Autodesk Inventor part; units mm, degrees
ref_plane "YZ Plane" through (0, 0, 0) normal (1, 0, 0) x (0, 1, 0)
ref_plane "XZ Plane" through (0, 0, 0) normal (0, 1, 0) x (-1, 0, 0)
ref_plane "XY Plane" through (0, 0, 0) normal (0, 0, 1) x (1, 0, 0)
sketch "DrumSketch" plane through (0, 0, 0) normal (0, 0, 1) x (1, 0, 0)
  line L0 (0, 8.12) -> (0, -9.52)
  line L1 (-7.84, 0) -> (7.84, 0)
  circle A0 centre (0, 0) radius 4.2
  line L2 (-2.7, -3) -> (2.7, -3)
  line L3 (2.7, 0) -> (2.7, -7)
  line L4 (2.7, -7) -> (-2.7, -7)
  line L5 (-2.7, -7) -> (-2.7, 0)
  circle A1 centre (0, 0) radius 5.6
  dimension "d0" = 8.4
  dimension "d1" = 5.4
  dimension "d2" = 7
  dimension "d3" = 4
  dimension "d6" = 11.2
sketch "BodySketch" plane through (0, 0, 0) normal (0, 1, 0) x (-1, 0, 0)
  line L0 (8, 16) -> (-8, 16)
  line L1 (-8, 16) -> (-8, -16)
  line L2 (-8, -16) -> (8, -16)
  line L3 (8, -16) -> (8, 16)
  line L4 (0, -38.6) -> (0, 25.1)
  line L5 (-11.2, 0) -> (11.2, 0)
  circle A0 centre (5.5, 13.5) radius 1.1
  circle A1 centre (5.5, 13.5) radius 1.65
  circle A2 centre (5.5, -13.5) radius 1.1
  circle A3 centre (5.5, -13.5) radius 1.65
  circle A4 centre (-5.5, 13.5) radius 1.1
  circle A5 centre (-5.5, 13.5) radius 1.65
  circle A6 centre (-5.5, -13.5) radius 1.65
  circle A7 centre (-5.5, -13.5) radius 1.1
  line L6 (7, -16) -> (7, -18)
  line L7 (7, -18) -> (6, -18)
  line L8 (6, -18) -> (8, -29.5)
  line L9 (8, -29.5) -> (-8, -29.5)
  line L10 (-8, -29.5) -> (-6, -18)
  line L11 (-6, -18) -> (-7, -18)
  line L12 (-7, -18) -> (-7, -16)
  line L13 (3.7, -29.5) -> (3.7, -16)
  line L14 (-3.7, -29.5) -> (-3.7, -16)
  line L15 (2.4888, -22.75) -> (1.2404, -22.75)
  circle A8 centre (5.5, 13.5) radius 1.75
  circle A9 centre (5.5, -13.5) radius 1.75
  circle A10 centre (-5.5, 13.5) radius 1.75
  circle A11 centre (-5.5, -13.5) radius 1.75
  point P0 (0, 0)
  point P1 (-8, 0)
  point P2 (0, 16)
  point P3 (8, 0)
  point P4 (0, -16)
  dimension "d4" = 16
  dimension "d5" = 32
  dimension "d15" = 3.3
  dimension "d16" = 2.2
  dimension "d17" = 2.5
  dimension "d18" = 2.5
  dimension "d23" = 16
  dimension "d24" = 12
  dimension "d25" = 14
  dimension "d26" = 2
  dimension "d28" = 11.5
  dimension "d29" = 7.4
  dimension "d37" = 6.75
  dimension "d38" = 6.75
  dimension "d39" = 22.75
  dimension "d40" = 3.5
extrude "MainBody" add sketch "BodySketch" against normal blind 8 contours L3 L5 L4 L0 | L4 L5 L1 L0 | L3 L2 L4 L5 | L4 L2 L1 L5 | A0 | A1 | A2 | A3 | A4 | A5 | A6 | A7 | A8 | A9 | A10 | A11
extrude "TrapConnector" add sketch "BodySketch" along normal blind 8.4 from surface at -8 contours L4 L9 L14 L2 | L2 L13 L9 L4 | L6 L7 L8 L9 L13 L2 | L14 L9 L10 L11 L12 L2
extrude "SliderChannel" cut sketch "DrumSketch" along normal through all both and the other way through all contours L1 L3 L2 L0 | L0 L2 L5 L1 | A1 L0 A0 L3 | L3 L4 L0 A1 | A1 L0 L4 L5 | L5 A0 L0 A1 | L2 L3 A0 L0 | L0 A0 L5 L2
extrude "TrapChannel" cut sketch "BodySketch" against normal blind 5.7 from surface at 0.4 contours L4 L9 L14 L2 | L2 L13 L9 L4
extrude "DrumChannel" cut sketch "DrumSketch" along normal mid plane 22 contours A1 L1 A0 L0 | L0 A0 L1 A1 | A0 L1 L0 | L0 L1 A0 | A1 L3 A0 L1 | L1 A0 L5 A1 | L1 L3 L2 L0 | L0 L2 L5 L1 | A0 L3 L1 | L1 L5 A0 | A1 L0 A0 L3 | L5 A0 L0 A1 | L2 L3 A0 L0 | L0 A0 L5 L2
extrude "DrumBearing" cut sketch "DrumSketch" along normal mid plane 24.4 contours A0 L1 L0 | L0 L1 A0 | L1 L3 L2 L0 | L0 L2 L5 L1 | A0 L3 L1 | L1 L5 A0 | L2 L3 A0 L0 | L0 A0 L5 L2
extrude "FixHoleTop" cut sketch "BodySketch" against normal through all contours A0 | A2 | A4 | A7
extrude "FixHoleMid" cut sketch "BodySketch" along normal blind 7 from surface at -8 contours A0 | A1 | A2 | A3 | A4 | A5 | A6 | A7
extrude "FixHoleBottom" cut sketch "BodySketch" along normal blind 4 from surface at -8 contours A0 | A1 | A2 | A3 | A4 | A5 | A6 | A7 | A8 | A9 | A10 | A11
chamfer "TrapEdgeChamfer" distance 0.5 angle 45 2 edges at (-8, -3.8, -29.5) (8, -3.8, -29.5)
equation "\"d23\" = LeverConnectTrapWidthBottom"
equation "\"d24\" = LeverConnectTrapWidthTop"
equation "\"d28\" = LeverConnectTrapDepth"
equation "\"d37\" = d38"
equation "\"d30\" = RailHeight"
equation "\"RHtmp\" = 8.4"
equation "\"RTtmp\" = 2"
properties part number "SwitchLeverUnit_LowerCase"
Geometry check sheet. Reference: the model listing, model coordinates, mm. A direction names the side the tool comes from. Round coordinates to 2 decimals unless told otherwise and drop trailing zeros. Loops run counter-clockwise (first coordinate to the right, second up) from the corner with the lowest first, then second, coordinate; pieces in that order, holes last. Notation, with made-up numbers: M -37.75,52.5 L -5.75,52.5 A21 cw -5.75,89.5 Z; hole C 86,-22 d9. An arc over 180 degrees is marked long. Return JSON: item names as keys, results as strings. Group by question number.
(1) Go/stop test with flat-tipped pins: pin 1 (5.5 mm diameter, centred on x = 5.5, z = 13.5, fed in from -Y); pin 2 (1 mm diameter, centred on x = -6, z = -13, fed in from -Y); pin 3 (5.5 mm diameter, centred on x = -5.5, z = 13.5, fed in from +Y); pin 4 (5 mm diameter, centred on y = -1, z = -23.5, fed in from -X). Record where each tip stops, or that it passes through.
(2) Section check C-C, the plane z = -23. Enter the section's corners in (x, y).
(3) Section check B-B, the plane z = -1.5. Enter the section's corners in (x, y), and give its area (3 significant figures).
(4) Scan lines: line 1 along Z through (x, y) = (-5.5, -0.6); line 2 along Z through (x, y) = (-5.5, -5.6); line 3 along X through (y, z) = (-3.3, 13.5). Record each from-to range of solid material in increasing order. Write a range as [from, to].
(5) Section check A-A, the plane z = 13.5. Give the number of separate pieces and of enclosed holes in the cut face, and give its area (3 significant figures).
(6) Mould release check, pull along Z, two halves, no side actions. Record for faces 1 (the face through (-5, 0.4, -23)), 2 (the face through (-4, -2, 11)): pulls with the +Z half, pulls with the -Z half, needs draft (parallel to the pull), parting line crosses it, or undercut.
(7) Set-up check for faces 3 (the face through (3, -1, 12.2)), 4 (the face through (6.97, -3.86, -23.58)), 5 (the face through (-7, -4, -17)), 6 (the face through (7, 0, 0)), 7 (the face through (-3.85, -2.52, 13.43)): record each of +Z, -Z, +X, -X, +Y, -Y from which the full face is reachable in a straight line by a thin tool's end or side.
Data:
{
 "1": {"pin 1": "y = -8", "pin 2": "y = -1", "pin 3": "y = 0", "pin 4": "x = -7.39"},
 "2": {"outline": "M -6.87,-8 L 6.87,-8 L 6.87,0.4 L 3.7,0.4 L 3.7,-5.3 L 2.7,-5.3 L 2.7,-7 L -2.7,-7 L -2.7,-5.3 L -3.7,-5.3 L -3.7,0.4 L -6.87,0.4 Z"},
 "3": {"outline": "M -8,-8 L 8,-8 L 8,0 L 5.6,0 A5.6 cw 2.7,-4.91 L 2.7,-7 L -2.7,-7 L -2.7,-4.91 A5.6 cw -5.6,0 L -8,0 Z", "area": "70.0 mm²"},
 "4": {"line 1": "[-29.5, -14.6], [-12.4, -11], [11, 12.4], [14.6, 16]", "line 2": "[-29.5, -15.25], [-11.75, 11.75], [15.25, 16]", "line 3": "[-8, -7.15], [-3.85, -2.7], [2.7, 3.85], [7.15, 8]"},
 "5": {"separate pieces": "3", "enclosed holes": "0", "area": "38.0 mm²"},
 "6": {"face 1": "needs draft", "face 2": "undercut"},
 "7": {"face 3": "+Y", "face 4": "+X, +Y, -Y", "face 5": "-X, +Y, -Y", "face 6": "+Z, +X, -X, +Y", "face 7": "-Y"}
}
